```python
from build123d import *

# Parameters (mm, degrees)
SZKIC1_W                                          = 230
SZKIC1_H                                          = 150
DODANIE_WYCI_GNI_CIE1_DEPTH                       = 5
POG_BIENIE_WALCOWE_POD_M3_RUB_Z_BEM_S_D           = 3.6
POG_BIENIE_WALCOWE_POD_M3_RUB_Z_BEM_S_DEPTH       = 6.7
POG_BIENIE_WALCOWE_POD_M3_RUB_Z_BEM_S_CBORE_D     = 7
POG_BIENIE_WALCOWE_POD_M3_RUB_Z_BEM_S_CBORE_DEPTH = 2.4
POG_BIENIE_WALCOWE_POD_M3_RUB_Z_BEM_S_TIP         = 1.081549114
POG_BIENIE_WALCOWE_POD_M3_RUB_Z_B_2_D             = 3.6
POG_BIENIE_WALCOWE_POD_M3_RUB_Z_B_2_DEPTH         = 6.7
POG_BIENIE_WALCOWE_POD_M3_RUB_Z_B_2_CBORE_D       = 7
POG_BIENIE_WALCOWE_POD_M3_RUB_Z_B_2_CBORE_DEPTH   = 2.4
POG_BIENIE_WALCOWE_POD_M3_RUB_Z_B_2_TIP           = 1.081549114
SZKIC7_W                                          = 10
SZKIC7_H                                          = 50
DODANIE_WYCI_GNI_CIE3_DEPTH                       = 7
OTWORY_USTALAJ_CE_4_0MM1_D                        = 4
OTWORY_USTALAJ_CE_4_0MM1_DEPTH                    = 6.7


with BuildPart() as part:
    # Szkic1 → Dodanie-wyciągnięcie1 (new body)
    with BuildSketch(Plane.XY):
        Rectangle(SZKIC1_W, SZKIC1_H)
    extrude(amount=DODANIE_WYCI_GNI_CIE1_DEPTH)

    # Pog_bienie walcowe pod M3 _rub_ z _bem s
    with Locations(Plane(origin=(0, 0, 0), x_dir=(-1, 0, 0), z_dir=(0, 0, -1))):
        with Locations((105, 37.5), (105, 0), (105, -37.5), (-105, 0), (-105, 37.5)):
            CounterBoreHole(POG_BIENIE_WALCOWE_POD_M3_RUB_Z_BEM_S_D / 2, POG_BIENIE_WALCOWE_POD_M3_RUB_Z_BEM_S_CBORE_D / 2, POG_BIENIE_WALCOWE_POD_M3_RUB_Z_BEM_S_CBORE_DEPTH, depth=POG_BIENIE_WALCOWE_POD_M3_RUB_Z_BEM_S_DEPTH)
            with Locations((0, 0, -(POG_BIENIE_WALCOWE_POD_M3_RUB_Z_BEM_S_DEPTH + POG_BIENIE_WALCOWE_POD_M3_RUB_Z_BEM_S_TIP / 2))):  # 118° drill point
                Cone(0, POG_BIENIE_WALCOWE_POD_M3_RUB_Z_BEM_S_D / 2, POG_BIENIE_WALCOWE_POD_M3_RUB_Z_BEM_S_TIP, mode=Mode.SUBTRACT)

    # Pog_bienie walcowe pod M3 _rub_ z _b 2
    with Locations(Plane(origin=(0, 0, 0), x_dir=(-1, 0, 0), z_dir=(0, 0, -1))):
        with Locations((-76.666666667, 70), (-38.333333337, 70), (-7e-09, 70), (38.333333323, 70), (76.666666653, 70)):
            CounterBoreHole(POG_BIENIE_WALCOWE_POD_M3_RUB_Z_B_2_D / 2, POG_BIENIE_WALCOWE_POD_M3_RUB_Z_B_2_CBORE_D / 2, POG_BIENIE_WALCOWE_POD_M3_RUB_Z_B_2_CBORE_DEPTH, depth=POG_BIENIE_WALCOWE_POD_M3_RUB_Z_B_2_DEPTH)
            with Locations((0, 0, -(POG_BIENIE_WALCOWE_POD_M3_RUB_Z_B_2_DEPTH + POG_BIENIE_WALCOWE_POD_M3_RUB_Z_B_2_TIP / 2))):  # 118° drill point
                Cone(0, POG_BIENIE_WALCOWE_POD_M3_RUB_Z_B_2_D / 2, POG_BIENIE_WALCOWE_POD_M3_RUB_Z_B_2_TIP, mode=Mode.SUBTRACT)

    # Szkic7 → Dodanie-wyciągnięcie3 (add)
    with BuildSketch(Plane.XY.offset(5)):
        with Locations((105, -45)):
            Rectangle(SZKIC7_W, SZKIC7_H)
    extrude(amount=DODANIE_WYCI_GNI_CIE3_DEPTH)

    # Otwory ustalające Ø4.0mm1
    with Locations(Plane.XZ.offset(70)):
        with Locations((105, 8.5)):
            Hole(OTWORY_USTALAJ_CE_4_0MM1_D / 2, depth=OTWORY_USTALAJ_CE_4_0MM1_DEPTH)


solid = part.part
```
CAD build for the part. Positions are in the model's coordinates, mm. A direction names the side the tool comes from. Coordinates: 2 decimals unless noted, no trailing zeros. Order: outer loops, then holes, each group sorted by start corner. A loop starts at its lowest first (then second) coordinate and runs counter-clockwise, first axis right, second up. Notation, with made-up numbers: (-37, -39.75) - (11, -39.75) arc R23 cw to (11, -14.75) - close; hole circle Ø5 at (53.5, 63). An arc over 180 degrees is marked (long way). Answer in a Markdown table with one row per item.
1. 3-axis set-ups, long thin cutter, end or side, ignore diameter. For faces 4 (the face through (-108.34, 38.55, 1.18)), 5 (the face through (-115, -1, 2)), 6 (the face through (110, -45, 8)), 7 (the face through (102.7, -70, 8.5)): which of +Z, -Z, +X, -X, +Y, -Y reach the whole face in a straight line?
Answer:
| item | result |
|---|---|
| face 4 | -Z |
| face 5 | +Z, -Z, -X, +Y, -Y |
| face 6 | +Z, +X, +Y, -Y |
| face 7 | +Z, +X, -X, -Y |
2. Slice it at B-B, the plane z = 8.5. List the corners of the cut face in (x, y), then the cut area to 3 significant figures.
Answer:
| item | result |
|---|---|
| outline | (100, -70) - (103, -70) - (103, -63.3) - (107, -63.3) - (107, -70) - (110, -70) - (110, -20) - (100, -20) - close |
| area | 473 mm² |
3. Drill centre lines: L1, parallel to Y at x = 105, z = 0.7; L2, parallel to X at y = 70, z = 3.9; L3, parallel to Y at x = -105, z = 1.55. Where is each one in solid material? Low to high. Write a range as from..to.
Answer:
| item | result |
|---|---|
| L1 | -75..-3.5, 3.5..34, 41..75 |
| L2 | -115..-78.47, -74.87..-40.13, -36.53..-1.8, 1.8..36.53, 40.13..74.87, 78.47..115 |
| L3 | -75..-41, -34..-3.5, 3.5..34, 41..75 |
4. Slice it at C-C, the plane x = 30. List the corners of the cut face in (y, z), then the cut area to 3 significant figures.
Answer:
| item | result |
|---|---|
| outline | (-75, 0) - (75, 0) - (75, 5) - (-75, 5) - close |
| area | 750 mm² |
5. Pull direction Y, two halves, no side cores. Call faces 1 (the face through (35.1, 68.66, 1.18)), 2 (the face through (-2, 75, 2)), 3 (the face through (-2, 1, 5)): +Y half, -Y half, draft (parallel to the pull), parting line (faces both ways), or undercut.
Answer:
| item | result |
|---|---|
| face 1 | undercut |
| face 2 | +Y half |
| face 3 | draft |
6. Slice it at A-A, the plane y = -26. List the corners of the cut face in (x, z).
Answer:
| item | result |
|---|---|
| outline | (-115, 0) - (115, 0) - (115, 5) - (110, 5) - (110, 12) - (100, 12) - (100, 5) - (-115, 5) - close |
7. Flat gauge pins, fed straight in: P1, Ø1.5, axis at y = -41, z = 8.5, coming from the +X side; P2, Ø3.5, axis at y = -42, z = 9, coming from the -X side; P3, Ø4, axis at x = 38.33, y = 70, coming from the -Z side. Where does each tip first touch, or does it go through?
Answer:
| item | result |
|---|---|
| P1 | x = 110 |
| P2 | x = 100 |
| P3 | z = 2.4 |
8. Slice it at D-D, the plane y = 58.5. List the corners of the cut face in (x, z), then the cut area to 3 significant figures.
Answer:
| item | result |
|---|---|
| outline | (-115, 0) - (115, 0) - (115, 5) - (-115, 5) - close |
| area | 1,150 mm² |
